Design review of the part shown in the three views and the two pictorial views. Dimensions are in mm from the part's minimum x, y and z. A direction names the side the tool comes from. Give positions to 0.01 mm unless a question says otherwise; leave off trailing zeros. Write each loop counter-clockwise with the first axis right and the second up, starting at its lowest first coordinate (ties: lowest second). Pieces come first, ordered by that corner, then holes. Notation, with made-up numbers: M -31.5,88.25 L 11.5,88.25 A16 ccw 11.5,112.25 Z; hole C 38,3 d6. An arc over 180 degrees is marked long. Write item = value, one per line.
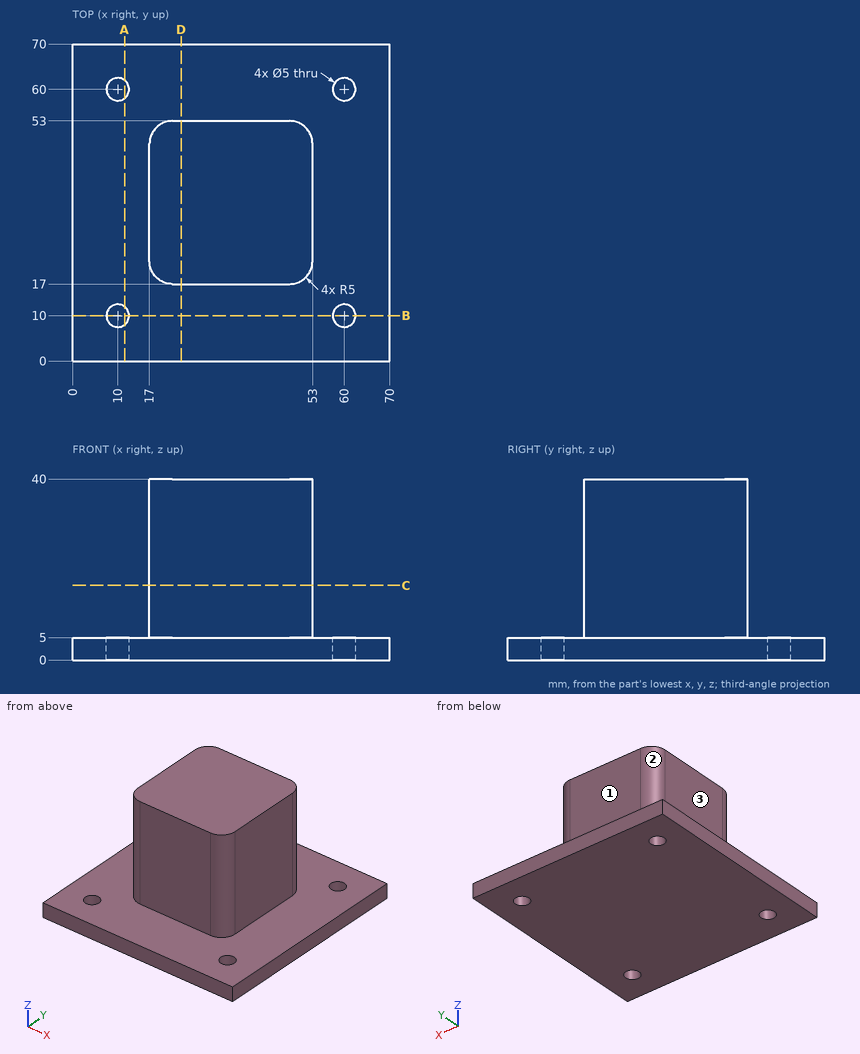
1. Machinability: for the marked faces 1, 2 and 3, which of the approach directions +Z, -Z, +X, -X, +Y, -Y give a long, thin tool a straight path to every point of the face, cutting with its end or side? Answer none if there is none.
Responses:
face_1 = +Z, +X, -X, +Y
face_2 = +Z, -X, +Y
face_3 = +Z, -X, +Y, -Y
2. We need section C-C, the plane z = 16.5. Write out the cut boundary in (x, y), then the cut area to 3 significant figures.
Responses:
outline = M 17,22 A5 ccw 22,17 L 48,17 A5 ccw 53,22 L 53,48 A5 ccw 48,53 L 22,53 A5 ccw 17,48 Z
area = 1,270 mm2
3. For line 1 along Y through (x, z) = (60, 3.75); line 2 along Y through (x, z) = (33, 5.5), list the stretches that pass through material, from the lowest coordinate up. Write a range as from..to.
Responses:
line_1 = 0..7.5, 12.5..57.5, 62.5..70
line_2 = 17..53
4. We need section B-B, the plane y = 10. Write out the cut boundary in (x, z), then the cut area to 3 significant figures.
Responses:
outline = M 0,0 L 7.5,0 L 7.5,5 L 0,5 Z; M 12.5,0 L 57.5,0 L 57.5,5 L 12.5,5 Z; M 62.5,0 L 70,0 L 70,5 L 62.5,5 Z
area = 300 mm2
5. We need section A-A, the plane x = 11.5. Write out the cut boundary in (y, z), then the cut area to 3 significant figures.
Responses:
outline = M 0,0 L 8,0 L 8,5 L 0,5 Z; M 12,0 L 58,0 L 58,5 L 12,5 Z; M 62,0 L 70,0 L 70,5 L 62,5 Z
area = 310 mm2
6. Insertion check: P1, Ø8, axis at x = 60, y = 10, coming from the -Z side; P2, Ø10, axis at y = 39, z = 11.5, coming from the -X side; P3, Ø4.5, axis at x = 10, y = 60, coming from the -Z side; P4, Ø2, axis at y = 21.5, z = 30.5, coming from the +X side. Each pin has a flat end and moves straight along its axis. Give the tip position at first contact, or say it passes through.
Responses:
P1 = 0
P2 = 17
P3 = through
P4 = 53
7. We need section D-D, the plane x = 24. Write out the cut boundary in (y, z), then the cut area to 3 significant figures.
Responses:
outline = M 0,0 L 70,0 L 70,5 L 53,5 L 53,40 L 17,40 L 17,5 L 0,5 Z
area = 1,610 mm2
